CAD build for the part. Positions are in the model's coordinates, mm. A direction names the side the tool comes from. Round coordinates to 2 decimals unless told otherwise and drop trailing zeros. Write each loop counter-clockwise with the first axis right and the second up, starting at its lowest first coordinate (ties: lowest second). Pieces come first, ordered by that corner, then holes. Notation, with made-up numbers: M 37.25,18 L 95.25,18 A18 cw 95.25,33 Z; hole C -27.5,23 d4. An arc over 180 degrees is marked long. Write each question's results on one line, items separated by ' | '. Start each with the question number.
```python
from build123d import *

# Parameters (mm, degrees)
F0_W     = 1600
F0_H     = 800
F1_DEPTH = 30
F2_W     = 30
F2_H     = 30
F3_DEPTH = 690


with BuildPart() as f1:
    # F0 (on Top) → F1 (new body)
    with BuildSketch(Plane.XY):
        with Locations((800, 400)):
            Rectangle(F0_W, F0_H)
    extrude(amount=F1_DEPTH)

    # F2 (on Top) → F3 (join)
    with BuildSketch(Plane.XY):
        with Locations((15, 15)):
            Rectangle(F2_W, F2_H)
        with Locations((15, 785)):
            Rectangle(F2_W, F2_H)
        with Locations((1585, 15)):
            Rectangle(F2_W, F2_H)
        with Locations((1585, 785)):
            Rectangle(F2_W, F2_H)
    extrude(amount=-F3_DEPTH)


solid = f1.part
```
1) Saw through at A-A, the plane z = -536.5. Write the cut outline in (x, y).
2) Saw through at C-C, the plane x = 1421.5. Write the cut outline in (y, z).
3) Pull direction X, two halves, no side cores. Call faces 4 (the face through (1570, 785, -340)), 5 (the face through (0, 398, 18)), 6 (the face through (789, 406, 30)): pulls with the +X half, pulls with the -X half, needs draft (parallel to the pull), parting line crosses it, or undercut.
4) Wall check: line 1 along Z through (x, y) = (1354.5, 556.5). Give the ranges that are in metal, low to high. Write a range as from..to.
5) Saw through at B-B, the plane y = 298. Write the cut outline in (x, z).
6) 3-axis set-ups, long thin cutter, end or side, ignore diameter. For faces 1 (the face through (15, 770, -340)), 2 (the face through (1585, 785, -690)), 3 (the face through (30, 15, -340)): which of +Z, -Z, +X, -X, +Y, -Y reach the whole face in a straight line?
Filled sheet:
1) outline: M 0,0 L 30,0 L 30,30 L 0,30 Z; M 0,770 L 30,770 L 30,800 L 0,800 Z; M 1570,0 L 1600,0 L 1600,30 L 1570,30 Z; M 1570,770 L 1600,770 L 1600,800 L 1570,800 Z
2) outline: M 0,0 L 800,0 L 800,30 L 0,30 Z
3) face 4: undercut | face 5: pulls with the -X half | face 6: needs draft
4) line 1: z = 0..30
5) outline: M 0,0 L 1600,0 L 1600,30 L 0,30 Z
6) face 1: -Z, +X, -X | face 2: -Z, +X, -X, +Y, -Y | face 3: -Z, +Y, -Y
